from build123d import *

# Parameters (mm, degrees)
BOSS_EXTRUDE1_DEPTH = 6.35
SKETCH2_R           = 10.0203
SKETCH2_R_2         = 1.8288
SKETCH2_W           = 19.05
SKETCH2_H           = 6.35
CUT_EXTRUDE1_DEPTH  = 131.484388434


with BuildPart() as part:
    # Sketch1 → Boss-Extrude1 (new body)
    with BuildSketch(Plane.XY):
        Polygon((-95.25, -3.175), (44.45, -3.175), (44.45, 3.175), (57.15, 3.175), (57.15, 9.525), (50.8, 9.525), (50.8, 60.325), (57.15, 60.325), (57.15, 66.675), (44.45, 66.675), (44.45, 73.025), (-95.25, 73.025), (-95.25, 66.675), (-107.95, 66.675), (-107.95, 60.325), (-101.6, 60.325), (-101.6, 9.525), (-107.95, 9.525), (-107.95, 3.175), (-95.25, 3.175), align=None)
    extrude(amount=BOSS_EXTRUDE1_DEPTH)

    # Sketch2 → Cut-Extrude1 (cut, through all)
    with BuildSketch(Plane.XY.offset(6.35)):
        with Locations((30.5689, 23.4061)):
            Circle(SKETCH2_R)
        with Locations((30.5689, 38.4061)):
            Circle(SKETCH2_R_2)
        with Locations((17.578518943, 15.9061)):
            Circle(SKETCH2_R_2)
        with Locations((43.559281057, 15.9061)):
            Circle(SKETCH2_R_2)
        with Locations((47.625, 57.15)):
            Rectangle(SKETCH2_W, SKETCH2_H)
        with Locations((-98.425, 57.15)):
            Rectangle(SKETCH2_W, SKETCH2_H)
    extrude(amount=-CUT_EXTRUDE1_DEPTH, mode=Mode.SUBTRACT)


solid = part.part
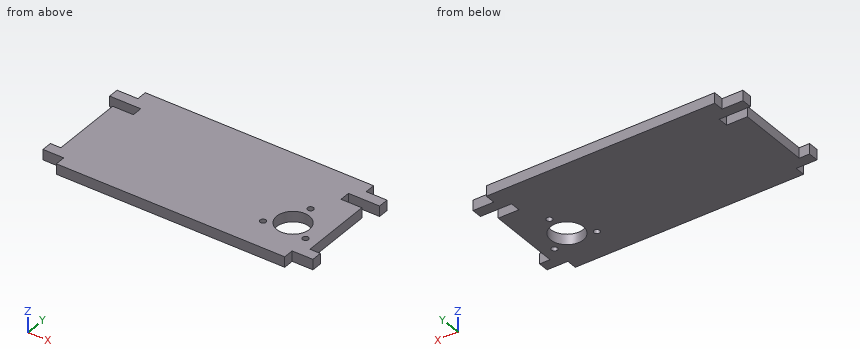
Check sheet for the modelled part. Datum: model origin and axes. Units: mm. Round coordinates to 2 decimals unless told otherwise and drop trailing zeros. Write each loop counter-clockwise with the first axis right and the second up, starting at its lowest first coordinate (ties: lowest second). Pieces come first, ordered by that corner, then holes. Notation, with made-up numbers: (63, 40.5) - (71, 40.5) arc R11 ccw to (71, 49.5) - close; hole circle Ø8 at (-21.75, 49). An arc over 180 degrees is marked (long way). Return JSON: item names as keys, results as strings.
Q1. Cross-section at A-A (z = 1.25). Record the boundary of the cut face in (x, y) (3 decimals), then the cut area to 3 significant figures.
Returned:
{"outline": "(-107.95, 3.175) - (-95.25, 3.175) - (-95.25, -3.175) - (44.45, -3.175) - (44.45, 3.175) - (57.15, 3.175) - (57.15, 9.525) - (50.8, 9.525) - (50.8, 53.975) - (38.1, 53.975) - (38.1, 60.325) - (57.15, 60.325) - (57.15, 66.675) - (44.45, 66.675) - (44.45, 73.025) - (-95.25, 73.025) - (-95.25, 66.675) - (-107.95, 66.675) - (-107.95, 60.325) - (-88.9, 60.325) - (-88.9, 53.975) - (-101.6, 53.975) - (-101.6, 9.525) - (-107.95, 9.525) - close; hole circle Ø3.658 at (17.579, 15.906); hole circle Ø20.041 at (30.569, 23.406); hole circle Ø3.658 at (30.569, 38.406); hole circle Ø3.658 at (43.559, 15.906)", "area": "11,100 mm²"}
Q2. Depth check by flat-ended pin: P1, Ø3, axis at y = 1, z = 3.5, coming from the +X side; P2, Ø1.9, axis at y = 37, z = 3.5, coming from the +X side; P3, Ø1.9, axis at x = 55.5, z = 2.5, coming from the +Y side (3 decimals). Enter the tip coordinate at first touch or a pass-through.
Returned:
{"P1": "stops at x = 44.45", "P2": "stops at x = 50.8", "P3": "stops at y = 66.675"}
Q3. Cross-section at B-B (y = 58). Record the boundary of the cut face in (x, z), then the cut area to 3 significant figures.
Returned:
{"outline": "(-88.9, 0) - (38.1, 0) - (38.1, 6.35) - (-88.9, 6.35) - close", "area": "806 mm²"}
Q4. Scan lines: L1, parallel to Y at x = 47, z = 6.25 (3 decimals); L2, parallel to X at y = 15, z = 6; L3, parallel to X at y = 53, z = 2.25. Record each from-to range of solid material in increasing order. Write a range as from..to.
Returned:
{"L1": "y = 3.175..53.975, 60.325..66.675", "L2": "x = -101.6..15.99, 19.17..25.12, 36.02..41.97, 45.15..50.8", "L3": "x = -101.6..50.8"}
